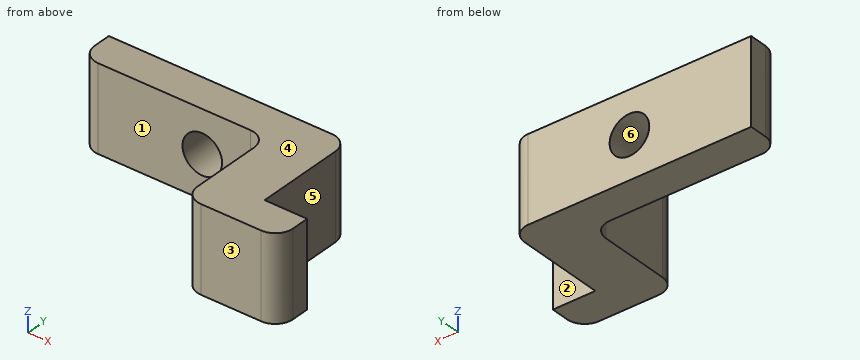
```python
from build123d import *

# Parameters (mm, degrees)
BOSS_EXTRUDE1_DEPTH = 7.62
SKETCH2_R           = 1.778
CUT_EXTRUDE1_DEPTH  = 27.181720723
FILLET1_R           = 1.5875


with BuildPart() as part:
    # Sketch1 → Boss-Extrude1 (new body)
    with BuildSketch(Plane.XY):
        Polygon((0, 0), (0, 9.525), (-21.59, 9.525), (-21.59, 6.35), (-4.7625, 6.35), (-4.7625, -3.175), (3.81, -3.175), (3.81, 0), align=None)
    extrude(amount=BOSS_EXTRUDE1_DEPTH)

    # Sketch2 → Cut-Extrude1 (cut, through all)
    with BuildSketch(Plane(origin=(0, 9.525, 0), x_dir=(1, 0, 0), z_dir=(0, 1, 0))):
        with Locations(Location((-10.668, -3.81, 0), (0, 0, 180))):
            Circle(SKETCH2_R)
    extrude(amount=-CUT_EXTRUDE1_DEPTH, mode=Mode.SUBTRACT)

    # Fillet1
    fillet1_edges = [part.edges().sort_by_distance(p)[0] for p in [
        (-4.7625, -3.175, 3.81),
        (-4.7625, 6.35, 3.81),
        (-21.59, 6.35, 3.81),
        (0, 9.525, 3.81),
        (3.81, -3.175, 3.81),
    ]]
    fillet(fillet1_edges, radius=FILLET1_R)


solid = part.part
```
For this review, take the finished solid that the model builds, in its own axes (mm). Face numbers are marked on the shaded views. A direction names the side the tool comes from. Round coordinates to 2 decimals unless told otherwise and drop trailing zeros. Order: outer loops, then holes, each group sorted by start corner. A loop starts at its lowest first (then second) coordinate and runs counter-clockwise, first axis right, second up.
Q1. Wall thickness on line 1 (Y direction, x = -18.5, z = 7) (3 decimals); line 2 (X direction, y = 8.25, z = 3.25); line 3 (X direction, y = 8, z = 7.25): over which ranges is each line inside the solid? List them lowest first.
Findings below:
line 1: y = 6.35 to 9.525
line 2: x = -21.59 to -12.36, -8.98 to -0.03
line 3: x = -21.59 to 0
Q2. Machinability: for the marked faces 1, 2 and 3, which of the approach directions +Z, -Z, +X, -X, +Y, -Y give a long, thin tool a straight path to every point of the face, cutting with its end or side? Answer none if there is none.
Findings below:
face 1: +Z, -Z, -X, -Y
face 2: +Z, -Z, +X, +Y
face 3: +Z, -Z, +X, -X, -Y
Q3. We need section C-C, the plane y = 7. Give the boundary of the cut face in (x, z), plus the area to 3 significant figures.
Findings below:
outline: (-21.28, 0) - (0, 0) - (0, 7.62) - (-21.28, 7.62) - close; hole circle Ø3.56 at (-10.67, 3.81)
area: 152 mm2
Q4. We need section D-D, the plane x = -14.5. Give the boundary of the cut face in (y, z) (3 decimals).
Findings below:
outline: (6.35, 0) - (9.525, 0) - (9.525, 7.62) - (6.35, 7.62) - close
Q5. Mouldability with a two-part tool opening along Z and no side actions: class the marked faces 4, 5 and 6 as pulls with the +Z half, pulls with the -Z half, needs draft (parallel to the pull), parting line crosses it, or undercut.
Findings below:
face 4: pulls with the +Z half
face 5: needs draft
face 6: undercut
Q6. Insertion check: P1, Ø1.5, axis at y = 4.5, z = 1.5, coming from the -X side; P2, Ø1, axis at x = -17, z = 3.5, coming from the -Y side; P3, Ø4, axis at y = 5, z = 3.5, coming from the +X side. Each pin has a flat end and moves straight along its axis. Give the tip position at first contact, or say it passes through.
Findings below:
P1: stops at x = -4.84
P2: stops at y = 6.35
P3: stops at x = 0
